The model under review builds one solid part; all positions refer to its coordinate system, in mm. Coordinates: 2 decimals unless noted, no trailing zeros. Order: outer loops, then holes, each group sorted by start corner. A loop starts at its lowest first (then second) coordinate and runs counter-clockwise, first axis right, second up. Notation, with made-up numbers: M 20.5,38 L 73.5,38 A29 ccw 73.5,77 Z; hole C 8.5,14.5 d3. An arc over 180 degrees is marked long. Answer as CSV lines item,"result". Start each with the question number.
Q1. Consider section D-D on z = 49. Write out the cut boundary in (x, y).
Q2. Wall thickness on L1, parallel to X at y = 3.2, z = 38; L2, parallel to X at y = 2.6, z = 18.5; L3, parallel to X at y = 3.6, z = 10.5: over which ranges is each line inside the solid? List them lowest first. Write a range as [from, to].
Q3. Consider section B-B on x = 27. Write out the cut boundary in (y, z), and give its area (3 significant figures).
Q4. Consider section C-C on x = 0. State how many separate pieces and enclosed holes the cut face has, and give its area (3 significant figures).
Q5. Consider section A-A on z = 35. Write out the cut boundary in (x, y), and give its area (3 significant figures).
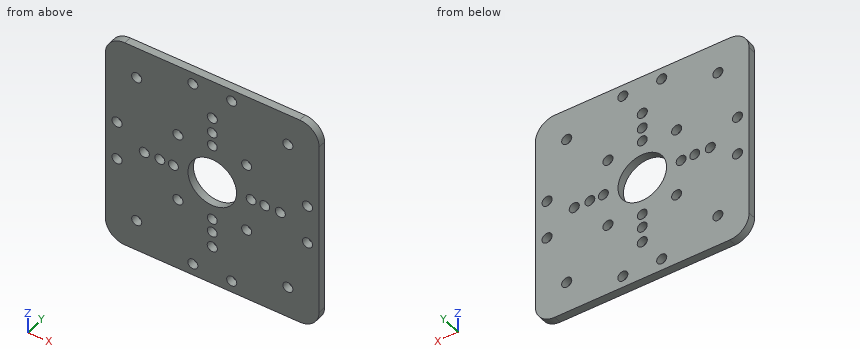
from build123d import *

# Parameters (mm, degrees)
SKETCH_1_W          = 110
SKETCH_1_H          = 110
EXTRUDE_1_DEPTH     = 4
SKETCH_2_R          = 2.6
CUT_EXTRUDE_1_DEPTH = 78.884529914
SKETCH_3_R          = 2.55
CUT_EXTRUDE_2_DEPTH = 78.884529914
SKETCH_4_R          = 2.6
CUT_EXTRUDE_3_DEPTH = 78.884529914
SKETCH_6_R          = 2.6
CUT_EXTRUDE_4_DEPTH = 10
SKETCH_7_R          = 2.6
CUT_EXTRUDE_5_DEPTH = 78.884529914
SKETCH_8_R          = 2.55
CUT_EXTRUDE_6_DEPTH = 78.884529914
SKETCH_9_R          = 12.5
CUT_EXTRUDE_7_DEPTH = 78.884529914
FILLET_1_R          = 10


with BuildPart() as part:
    # 草图1 → 凸台-拉伸1 (new body)
    with BuildSketch(Plane(origin=(0, 0, 0), x_dir=(1, 0, 0), z_dir=(0, 1, 0))):
        Rectangle(SKETCH_1_W, SKETCH_1_H)
    extrude(amount=EXTRUDE_1_DEPTH)

    # 草图2 → 切除-拉伸1 (cut, through all)
    with BuildSketch(Plane(origin=(0, 0, 0), x_dir=(1, 0, 0), z_dir=(0, 1, 0))):
        with Locations(Location((0, 35, 0), (0, 0, 270))):
            Circle(SKETCH_2_R)
        with Locations(Location((35, 0, 0), (0, 0, 270))):
            Circle(SKETCH_2_R)
        with Locations(Location((0, -35, 0), (0, 0, 270))):
            Circle(SKETCH_2_R)
        with Locations(Location((-35, 0, 0), (0, 0, 270))):
            Circle(SKETCH_2_R)
    extrude(amount=CUT_EXTRUDE_1_DEPTH, mode=Mode.SUBTRACT)

    # 草图3 → 切除-拉伸2 (cut, through all)
    with BuildSketch(Plane(origin=(0, 4, 0), x_dir=(1, 0, 0), z_dir=(0, 1, 0))):
        with Locations(Location((0, 27, 0), (0, 0, 270))):
            Circle(SKETCH_3_R)
        with Locations(Location((27, 0, 0), (0, 0, 270))):
            Circle(SKETCH_3_R)
        with Locations(Location((0, -27, 0), (0, 0, 270))):
            Circle(SKETCH_3_R)
        with Locations(Location((-27, 0, 0), (0, 0, 270))):
            Circle(SKETCH_3_R)
    extrude(amount=-CUT_EXTRUDE_2_DEPTH, mode=Mode.SUBTRACT)

    # 草图4 → 切除-拉伸3 (cut, through all)
    with BuildSketch(Plane(origin=(0, 4, 0), x_dir=(1, 0, 0), z_dir=(0, 1, 0))):
        with Locations(Location((-10, 49, 0), (0, 0, 270))):
            Circle(SKETCH_4_R)
        with Locations(Location((10, 49, 0), (0, 0, 270))):
            Circle(SKETCH_4_R)
        with Locations(Location((49, 10, 0), (0, 0, 270))):
            Circle(SKETCH_4_R)
        with Locations(Location((49, -10, 0), (0, 0, 270))):
            Circle(SKETCH_4_R)
        with Locations(Location((10, -49, 0), (0, 0, 270))):
            Circle(SKETCH_4_R)
        with Locations(Location((-10, -49, 0), (0, 0, 270))):
            Circle(SKETCH_4_R)
        with Locations(Location((-49, -10, 0), (0, 0, 270))):
            Circle(SKETCH_4_R)
        with Locations(Location((-49, 10, 0), (0, 0, 270))):
            Circle(SKETCH_4_R)
    extrude(amount=-CUT_EXTRUDE_3_DEPTH, mode=Mode.SUBTRACT)

    # 草图6 → 切除-拉伸4 (cut)
    with BuildSketch(Plane(origin=(0, 4, 0), x_dir=(1, 0, 0), z_dir=(0, 1, 0))):
        with Locations(Location((-38.890872965, 38.890872965, 0), (0, 0, 270))):
            Circle(SKETCH_6_R)
        with Locations(Location((38.890872965, 38.890872965, 0), (0, 0, 270))):
            Circle(SKETCH_6_R)
        with Locations(Location((38.890872965, -38.890872965, 0), (0, 0, 270))):
            Circle(SKETCH_6_R)
        with Locations(Location((-38.890872965, -38.890872965, 0), (0, 0, 270))):
            Circle(SKETCH_6_R)
    extrude(amount=-CUT_EXTRUDE_4_DEPTH, mode=Mode.SUBTRACT)

    # 草图7 → 切除-拉伸5 (cut, through all)
    with BuildSketch(Plane(origin=(0, 4, 0), x_dir=(1, 0, 0), z_dir=(0, 1, 0))):
        with Locations(Location((-17.67766953, 17.67766953, 0), (0, 0, 270))):
            Circle(SKETCH_7_R)
        with Locations(Location((17.67766953, 17.67766953, 0), (0, 0, 270))):
            Circle(SKETCH_7_R)
        with Locations(Location((17.67766953, -17.67766953, 0), (0, 0, 270))):
            Circle(SKETCH_7_R)
        with Locations(Location((-17.67766953, -17.67766953, 0), (0, 0, 270))):
            Circle(SKETCH_7_R)
    extrude(amount=-CUT_EXTRUDE_5_DEPTH, mode=Mode.SUBTRACT)

    # 草图8 → 切除-拉伸6 (cut, through all)
    with BuildSketch(Plane(origin=(0, 4, 0), x_dir=(1, 0, 0), z_dir=(0, 1, 0))):
        with Locations(Location((0, 20, 0), (0, 0, 270))):
            Circle(SKETCH_8_R)
        with Locations(Location((20, 0, 0), (0, 0, 270))):
            Circle(SKETCH_8_R)
        with Locations(Location((0, -20, 0), (0, 0, 270))):
            Circle(SKETCH_8_R)
        with Locations(Location((-20, 0, 0), (0, 0, 270))):
            Circle(SKETCH_8_R)
    extrude(amount=-CUT_EXTRUDE_6_DEPTH, mode=Mode.SUBTRACT)

    # 草图9 → 切除-拉伸7 (cut, through all)
    with BuildSketch(Plane(origin=(0, 4, 0), x_dir=(1, 0, 0), z_dir=(0, 1, 0))):
        with Locations(Location((0, 0, 0), (0, 0, 270))):
            Circle(SKETCH_9_R)
    extrude(amount=-CUT_EXTRUDE_7_DEPTH, mode=Mode.SUBTRACT)

    # 圆角1
    fillet_1_edges = [part.edges().sort_by_distance(p)[0] for p in [
        (55, 2, 55),
        (-55, 2, 55),
        (-55, 2, -55),
        (55, 2, -55),
    ]]
    fillet(fillet_1_edges, radius=FILLET_1_R)


solid = part.part
Evaluation:
1,outline,"M -54.17,0 L -12.6,0 L -12.6,4 L -54.17,4 Z; M -7.4,0 L 7.4,0 L 7.4,4 L -7.4,4 Z; M 12.6,0 L 54.17,0 L 54.17,4 L 12.6,4 Z"
2,L1,"x = [-55, -41.33], [-36.45, 36.45], [41.33, 55]"
2,L2,"x = [-55, -20.14], [-15.21, -2.06], [2.06, 15.21], [20.14, 55]"
2,L3,"x = [-55, -51.55], [-46.45, -6.78], [6.78, 46.45], [51.55, 55]"
3,outline,"M 0,-55 L 4,-55 L 4,-2.55 L 0,-2.55 Z; M 0,2.55 L 4,2.55 L 4,55 L 0,55 Z"
3,area,"420 mm²"
4,separate pieces,"8"
4,enclosed holes,"0"
4,area,"217 mm²"
5,outline,"M -55,0 L -2.6,0 L -2.6,4 L -55,4 Z; M 2.6,0 L 55,0 L 55,4 L 2.6,4 Z"
5,area,"419 mm²"
